For this review, use the dimensioned drawing (mm, ordinates from the lowest corner) and the shaded views. Give positions to 0.01 mm unless a question says otherwise; leave off trailing zeros. Order: outer loops, then holes, each group sorted by start corner. A loop starts at its lowest first (then second) coordinate and runs counter-clockwise, first axis right, second up. Notation, with made-up numbers: (48, -38) -> (99, -38) arc R31 cw to (99, -12) -> close; hole circle Ø7 at (-13, 13.25). An arc over 180 degrees is marked (long way). One line per item, written item: value. Start each with the question number.
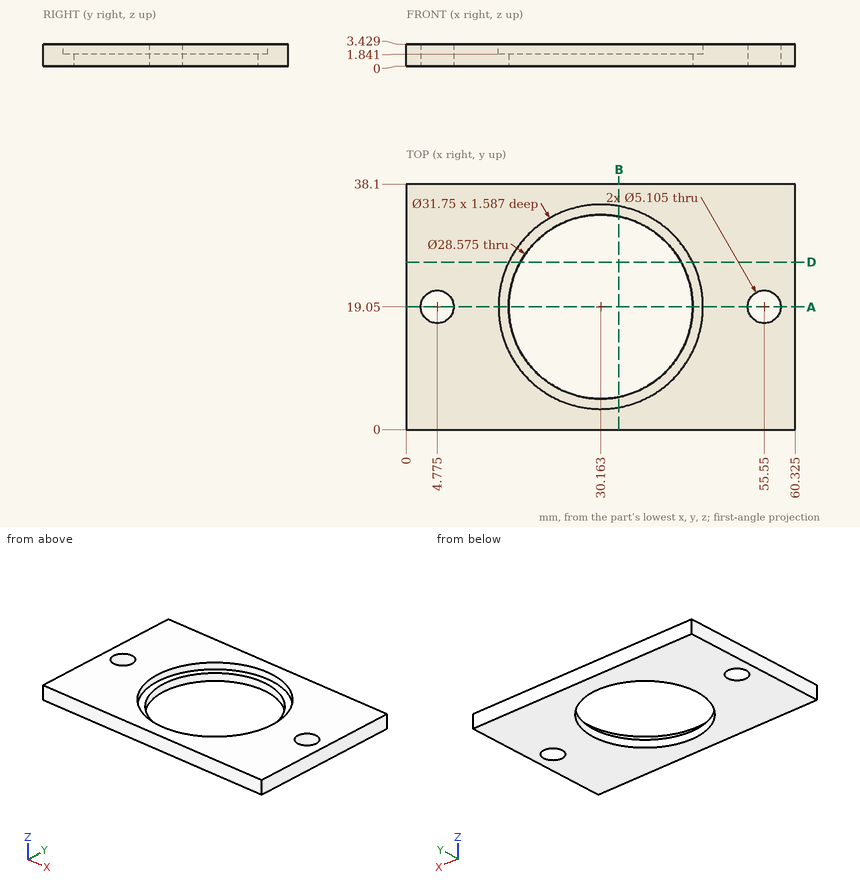
Q1. Take a section at B-B (x = 33). State the section outline as (y, z) points.
Q2. Take a section at D-D (y = 26). State the section outline as (x, z) points (1 decimal).
Q3. For line 1 along X through (y, z) = (19, 2.4) (1 decimal); line 2 along Y through (x, z) = (30.5, 0.55); line 3 along X through (y, z) = (6.5, 0.5) (1 decimal), list the stretches that pass through material, from the lowest coordinate up.
Q4. Take a section at A-A (y = 19.05). State how many separate pieces and enclosed holes the cut face has.
Q5. For pin 1 Ø6.5 at (x, y) = (55.55, 19.05) entering from -Z, flat-tipped, find the tip position at first contact; note if it passes through.
Answers below:
1. outline: (0, 0) -> (5.05, 0) -> (5.05, 1.84) -> (3.43, 1.84) -> (3.43, 3.43) -> (0, 3.43) -> close; (33.05, 0) -> (38.1, 0) -> (38.1, 3.43) -> (34.67, 3.43) -> (34.67, 1.84) -> (33.05, 1.84) -> close
2. outline: (0, 0) -> (17.7, 0) -> (17.7, 1.8) -> (15.9, 1.8) -> (15.9, 3.4) -> (0, 3.4) -> close; (42.6, 0) -> (60.3, 0) -> (60.3, 3.4) -> (44.4, 3.4) -> (44.4, 1.8) -> (42.6, 1.8) -> close
3. line 1: x = 0 to 2.2, 7.3 to 14.3, 46 to 53, 58.1 to 60.3
3. line 2: y = 0 to 4.77, 33.33 to 38.1
3. line 3: x = 0 to 23.3, 37 to 60.3
4. separate pieces: 4
4. enclosed holes: 0
5. pin 1: stops at z = 0
